```python
from build123d import *

# Parameters (mm, degrees)
BOSS_EXTRUDE1_DEPTH   = 0.75438
ESBO_O1_R             = 1.09200001
CORTE_EXTRUS_O1_DEPTH = 10


with BuildPart() as part:
    # Sketch1 → Boss-Extrude1 (new body)
    with BuildSketch(Plane.XY):
        with BuildLine():
            Line((-15, -35), (15, -35))
            Line((15, -35), (26.292884648, -14.44590658))
            ThreePointArc((26.292884648, -14.44590658), (0, 30), (-26.292884648, -14.44590658))
            Line((-26.292884648, -14.44590658), (-15, -35))
        make_face()
    extrude(amount=BOSS_EXTRUDE1_DEPTH)

    # Esboço1 → Corte-extrusão1 (cut)
    with BuildSketch(Plane.XY.offset(0.75438)):
        with Locations((-7.4931, -32.938)):
            Circle(ESBO_O1_R)
        with Locations((-7.366, 26.4469878)):
            Circle(ESBO_O1_R)
        with Locations((-27.559, -0.0450022)):
            Circle(ESBO_O1_R)
        with Locations((-19.634, -19.9840012)):
            Circle(ESBO_O1_R)
        with Locations((7.366, 26.4469878)):
            Circle(ESBO_O1_R)
        with Locations((7.4931, -32.938)):
            Circle(ESBO_O1_R)
        with Locations((19.634, -19.9840012)):
            Circle(ESBO_O1_R)
        with Locations((27.559, -0.0450022)):
            Circle(ESBO_O1_R)
    extrude(amount=-CORTE_EXTRUS_O1_DEPTH, mode=Mode.SUBTRACT)


solid = part.part
```
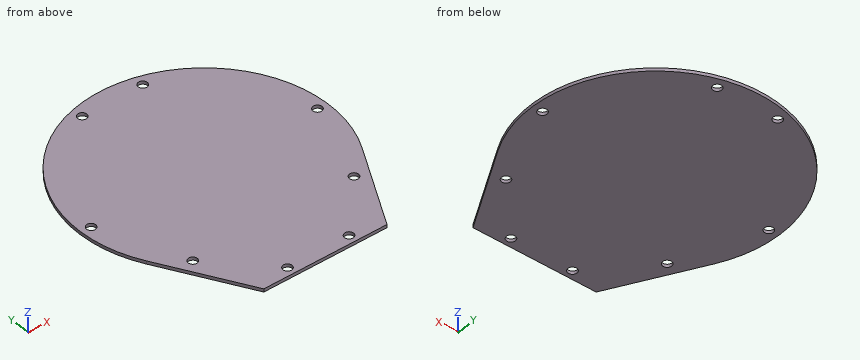
Work out the finished part from the listing and answer in its coordinate system (mm). Coordinates: 2 decimals unless noted, no trailing zeros. Loops run counter-clockwise (first coordinate to the right, second up) from the corner with the lowest first, then second, coordinate; pieces in that order, holes last.
1) Section D-D (x = -11.5) is taken. Give the vertices of the cut face in (y, z).
Results:
outline: (-35, 0) - (27.71, 0) - (27.71, 0.75) - (-35, 0.75) - close
2) Section B-B (x = -20) is taken. Give the vertices of the cut face in (y, z), plus the area to 3 significant figures.
Results:
outline: (-25.9, 0) - (-21.01, 0) - (-21.01, 0.75) - (-25.9, 0.75) - close; (-18.96, 0) - (22.36, 0) - (22.36, 0.75) - (-18.96, 0.75) - close
area: 34.9 mm2
3) Section C-C (y = -26.5) is taken. Give the vertices of the cut face in (x, z).
Results:
outline: (-19.67, 0) - (19.67, 0) - (19.67, 0.75) - (-19.67, 0.75) - close
4) A flat-ended cylindrical pin translates along its axis: pin 1 (1.7 mm diameter, centred on x = 7.37, y = 26.45, fed in from +Z). Find the tip coordinate at first contact, or state that the pin passes through.
Results:
pin 1: passes through
5) Consider probe 1 along Y at (x, z) = (-19, 0.2); probe 2 along Y at (x, z) = (20, 0.1); probe 3 along X at (y, z) = (12.5, 0.15). Determine where each line is inside the solid, lowest interval first.
Results:
probe 1: y = -27.72 to -20.87, -19.09 to 23.22
probe 2: y = -25.9 to -21.01, -18.96 to 22.36
probe 3: x = -27.27 to 27.27
6) Section A-A (z = 0.45) is taken. Give the number of separate pieces and of enclosed holes in the cut face, plus the area to 3 significant figures.
Results:
separate pieces: 1
enclosed holes: 8
area: 3,060 mm2
